Can you work these out from the model? Positions are in its coordinate system, mm. Coordinates: 2 decimals unless noted, no trailing zeros. Order: outer loops, then holes, each group sorted by start corner. A loop starts at its lowest first (then second) coordinate and runs counter-clockwise, first axis right, second up. Notation, with made-up numbers: (-30.5, 73) -> (2.5, 73) arc R23 ccw to (2.5, 82) -> close; hole circle Ø10 at (-38.75, 63.25). An arc over 180 degrees is marked (long way). Answer as a JSON object with one key per item and string values. Group by question number.
(1) If we mould it in two halves opening along X, with no side actions, what happens to faces 1 (the cylindrical face through (-0.7, -144.71, 2.19)), 2 (the flat face through (21.501, 95.732, 2.191)), 3 (the cylindrical face through (-2.38, 76.84, 2.19)), 4 (the cylindrical face through (-23.273, 83.094, 2.191))? For each: pulls with the +X half, pulls with the -X half, needs draft (parallel to the pull), parting line crosses it, or undercut.
(2) I want a section at B-B, the plane x = -16. List the corners of the cut face in (y, z) for me (3 decimals), plus the area to 3 significant figures.
(3) I want a section at D-D, the plane y = -3.5. List the corners of the cut face in (x, z) for me (3 decimals), plus the area to 3 significant figures.
(4) For pin 1 (5 mm diameter, centred on x = 0, y = 65.98, fed in from -Z); pin 2 (1.5 mm diameter, centred on x = 7, z = 3, fed in from +Y), each with a flat end and sliding along its axis, tell me the tip position at first contact or that it passes through.
(5) I want a section at C-C, the plane z = 2.35. State how many separate pieces and enclosed holes the cut face has, plus the area to 3 significant figures.
(6) I want a section at A-A, the plane x = 0. List the corners of the cut face in (y, z) for me (1 decimal), plus the area to 3 significant figures.
(7) I need wall thicknesses on line 1 (Y direction, x = -0.5, z = 1.2); line 2 (Y direction, x = 0, z = 2); line 3 (Y direction, x = -5, z = 3.9). Which ranges of each line are inside material? Lowest first, please.
from build123d import *

# Parameters (mm, degrees)
SKETCH2_R           = 23.0378
SKETCH2_R_2         = 3.175
SKETCH2_R_3         = 10.9855
BOSS_EXTRUDE1_DEPTH = 4.445
SKETCH4_R           = 3.175
CUT_EXTRUDE2_DEPTH  = 149.225118982
CUT_EXTRUDE3_DEPTH  = 149.225118982


with BuildPart() as part:
    # Sketch2 → Boss-Extrude1 (new body)
    with BuildSketch(Plane.XY):
        with BuildLine():
            Line((31.75, 112.9665), (-31.75, 112.9665))
            Line((-31.75, 112.9665), (-31.75, 53.2765))
            ThreePointArc((-31.75, 53.2765), (-12.7, -17.145), (-31.75, -87.5665))
            Line((-31.75, -87.5665), (-31.75, -112.9665))
            ThreePointArc((-31.75, -112.9665), (0, -144.7165), (31.75, -112.9665))
            Line((31.75, -112.9665), (31.75, -87.5665))
            ThreePointArc((31.75, -87.5665), (12.7, -17.145), (31.75, 53.2765))
            Line((31.75, 53.2765), (31.75, 112.9665))
        make_face()
        with Locations((0, -112.9665)):
            Circle(SKETCH2_R, mode=Mode.SUBTRACT)
        with Locations((-22.86, 79.9465)):
            Circle(SKETCH2_R_2, mode=Mode.SUBTRACT)
        with Locations((0, 65.9765)):
            Circle(SKETCH2_R_2, mode=Mode.SUBTRACT)
        with Locations((0, 87.5665)):
            Circle(SKETCH2_R_3, mode=Mode.SUBTRACT)
        with Locations((22.86, 79.9465)):
            Circle(SKETCH2_R_2, mode=Mode.SUBTRACT)
    extrude(amount=BOSS_EXTRUDE1_DEPTH)

    # Sketch4 → Cut-Extrude2 (cut, through all)
    with BuildSketch(Plane.XY.offset(4.445)):
        with Locations((0, 43.1165)):
            Circle(SKETCH4_R)
        with Locations((0, -50.419)):
            Circle(SKETCH4_R)
    extrude(amount=-CUT_EXTRUDE2_DEPTH, mode=Mode.SUBTRACT)

    # Sketch6 → Cut-Extrude3 (cut, through all)
    with BuildSketch(Plane(origin=(0, 0, 0), x_dir=(-1, 0, 0), z_dir=(0, 0, -1))):
        with BuildLine():
            Line((-31.75, 112.9665), (-31.75, 88.521600063))
            Line((-31.75, 88.521600063), (-10.961308866, 103.147007307))
            ThreePointArc((-10.961308866, 103.147007307), (0.491450562, 106.610159741), (11.750340751, 102.560898695))
            Line((11.750340751, 102.560898695), (31.75, 86.888192115))
            Line((31.75, 86.888192115), (31.75, 112.9665))
            Line((31.75, 112.9665), (-31.75, 112.9665))
        make_face()
    extrude(amount=-CUT_EXTRUDE3_DEPTH, mode=Mode.SUBTRACT)


solid = part.part
Computed values:
{
 "1": {"face 1": "parting line crosses it", "face 2": "pulls with the +X half", "face 3": "undercut", "face 4": "undercut"},
 "2": {"outline": "(-140.39, 0) -> (-129.542, 0) -> (-129.542, 4.445) -> (-140.39, 4.445) -> close; (-96.391, 0) -> (-47.329, 0) -> (-47.329, 4.445) -> (-96.391, 4.445) -> close; (13.039, 0) -> (99.231, 0) -> (99.231, 4.445) -> (13.039, 4.445) -> close", "area": "649 mm2"},
 "3": {"outline": "(-13.368, 0) -> (13.368, 0) -> (13.368, 4.445) -> (-13.368, 4.445) -> close", "area": "119 mm2"},
 "4": {"pin 1": "passes through", "pin 2": "stops at y = 105.56"},
 "5": {"separate pieces": "1", "enclosed holes": "7", "area": "9,200 mm2"},
 "6": {"outline": "(-144.7, 0) -> (-136, 0) -> (-136, 4.4) -> (-144.7, 4.4) -> close; (-89.9, 0) -> (-53.6, 0) -> (-53.6, 4.4) -> (-89.9, 4.4) -> close; (-47.2, 0) -> (39.9, 0) -> (39.9, 4.4) -> (-47.2, 4.4) -> close; (46.3, 0) -> (62.8, 0) -> (62.8, 4.4) -> (46.3, 4.4) -> close; (69.2, 0) -> (76.6, 0) -> (76.6, 4.4) -> (69.2, 4.4) -> close; (98.6, 0) -> (106.6, 0) -> (106.6, 4.4) -> (98.6, 4.4) -> close", "area": "730 mm2"},
 "7": {"line 1": "y = -144.71 to -136, -89.93 to -53.55, -47.28 to 39.98, 46.25 to 62.84, 69.11 to 76.59, 98.54 to 106.61", "line 2": "y = -144.72 to -136, -89.93 to -53.59, -47.24 to 39.94, 46.29 to 62.8, 69.15 to 76.58, 98.55 to 106.62", "line 3": "y = -144.32 to -135.46, -90.48 to 77.78, 97.35 to 105.95"}
}
